The figure shows three views and two pictorial views of one solid part (mm, origin at its lowest corner). Answer the questions. A direction names the side the tool comes from. Coordinates: 2 decimals unless noted, no trailing zeros. Order: outer loops, then holes, each group sorted by start corner. A loop starts at its lowest first (then second) coordinate and runs counter-clockwise, first axis right, second up. Notation, with made-up numbers: (77.5, 12.25) -> (102.5, 12.25) arc R18 ccw to (102.5, 43.25) -> close; hole circle Ø10 at (-3, 26.25). An arc over 180 degrees is marked (long way). Write item = value, one per line. Start each with the question number.
Q1. Straight lines are drawn through the part: L1, parallel to X at y = 12.5, z = 3; L2, parallel to Y at x = 52, z = 2; L3, parallel to Y at x = 33.5, z = 9. For each, find the intervals that lie inside material, in ascending order. Write a range as from..to.
Q2. The part is cut by section C-C, the plane z = 1. Determine the outline of the cut face in (x, y), plus the area to 3 significant figures.
Q3. For a pull along X with two mould halves and no side action, classify the marked faces 1, 2 and 3 as +X half, -X half, draft (parallel to the pull), parting line (faces both ways), or undercut.
Q4. Flat-ended cylindrical pins translate along their axes: pin 1 (1.6 mm diameter, centred on y = 0.5, z = 5.5, fed in from +X); pin 2 (1.6 mm diameter, centred on x = 28.5, y = 1, fed in from -Z); pin 3 (6 mm diameter, centred on x = 17.5, z = 4, fed in from -Y); pin 4 (6 mm diameter, centred on x = 30, y = 16, fed in from -Z). Find the tip coordinate at first contact, or state that the pin passes through.
Q5. The part is cut by section B-B, the plane x = 48.5. Determine the outline of the cut face in (y, z), plus the area to 3 significant figures.
Q6. The part is cut by section D-D, the plane z = 6.5. Determine the outline of the cut face in (x, y).
Q7. The part is cut by section A-A, the plane y = 18.25. Determine the outline of the cut face in (x, z).
Q8. Which of the six approach directions +Z, -Z, +X, -X, +Y, -Y give full straight-line access (tool end or side, diameter ignored) to the marked faces 4, 5 and 6?
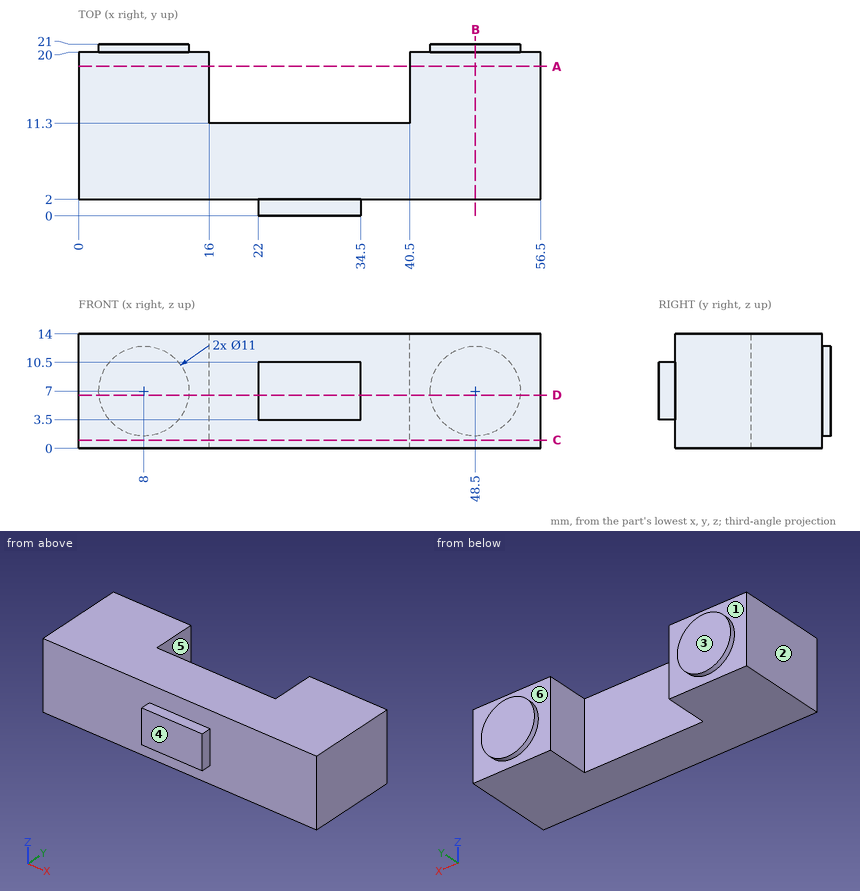
Model answer:
q1.L1 = 0..16, 40.5..56.5
q1.L2 = 2..20
q1.L3 = 0..11.3
q2.outline = (0, 2) -> (56.5, 2) -> (56.5, 20) -> (40.5, 20) -> (40.5, 11.3) -> (16, 11.3) -> (16, 20) -> (0, 20) -> close
q2.area = 804 mm2
q3.face_1 = undercut
q3.face_2 = -X half
q3.face_3 = draft
q4.pin_1 = 34.5
q4.pin_2 = 3.5
q4.pin_3 = 2
q4.pin_4 = through
q5.outline = (2, 0) -> (20, 0) -> (20, 1.5) -> (21, 1.5) -> (21, 12.5) -> (20, 12.5) -> (20, 14) -> (2, 14) -> close
q5.area = 263 mm2
q6.outline = (0, 2) -> (22, 2) -> (22, 0) -> (34.5, 0) -> (34.5, 2) -> (56.5, 2) -> (56.5, 20) -> (53.98, 20) -> (53.98, 21) -> (43.02, 21) -> (43.02, 20) -> (40.5, 20) -> (40.5, 11.3) -> (16, 11.3) -> (16, 20) -> (13.48, 20) -> (13.48, 21) -> (2.52, 21) -> (2.52, 20) -> (0, 20) -> close
q7.outline = (0, 0) -> (16, 0) -> (16, 14) -> (0, 14) -> close; (40.5, 0) -> (56.5, 0) -> (56.5, 14) -> (40.5, 14) -> close
q8.face_4 = +Z, -Z, +X, -X, -Y
q8.face_5 = +Z, -Z, +Y
q8.face_6 = +Y
